Source: CAD feature listing. Evaluate the final solid. Frame: model axes, mm. Coordinates: 2 decimals unless noted, no trailing zeros. Write each loop counter-clockwise with the first axis right and the second up, starting at its lowest first coordinate (ties: lowest second). Pieces come first, ordered by that corner, then holes. Notation, with made-up numbers: M 21.25,-17.75 L 31.25,-17.75 A14 cw 31.25,7.25 Z; hole C 65.25,-20 d8. An arc over 180 degrees is marked long. One line per item, written item: value. Start each with the question number.
Item 1: Mould query, pull axis Z, two halves, no side actions, for faces 1 (the flat face through (7, 3, -1.9)), 2 (the flat face through (60, 3, 0)), 3 (the flat face through (94, 3, -6.1)). Classes: released by +Z, released by -Z, zero draft, split by the parting line, or undercut.
Item 2: Cut plane D-D, the plane x = 58. Output: boundary loops of the cut face in (y, z), then the cut area to 3 significant figures.
Item 3: Cut plane B-B, the plane z = -115. Output: boundary loops of the cut face in (x, y).
Item 4: Ray query, L1, parallel to Z at x = 43, y = 3.85; L2, parallel to Z at x = 106.2, y = 2.45; L3, parallel to X at y = 4.75, z = -115. Return the intervals inside material, ascending. Write a range as from..to.
Item 5: Pin query (flat end, axial travel): P1, Ø3, axis at x = 57.5, z = -30.5, coming from the +Y side. Return the tip coordinate at first contact, or that it passes through.
Item 6: Cut plane C-C, the plane z = -31.5. Output: boundary loops of the cut face in (x, y), then the cut area to 3 significant figures.
Item 7: Cut plane A-A, the plane x = 15.2. Output: boundary loops of the cut face in (y, z).
```python
from build123d import *

# Parameters (mm, degrees)
SKETCH_1_W          = 121.4
SKETCH_1_H          = 128.7
EXTRUDE_1_DEPTH     = 1.5
EXTRUDE_2_DEPTH     = 2
SKETCH_3_W          = 1.5
SKETCH_3_H          = 96.8
SKETCH_3_W_2        = 113.8
SKETCH_3_H_2        = 1.5
EXTRUDE_3_DEPTH     = 2
SKETCH_5_W          = 121.4
SKETCH_5_H          = 8
SKETCH_5_W_2        = 32.9
SKETCH_5_H_2        = 4.2
SKETCH_5_W_3        = 48
EXTRUDE_5_DEPTH     = 4
SKETCH_7_R          = 4.75
EXTRUDE_10_DEPTH    = 4
SKETCH_8_R          = 1.75
CUT_EXTRUDE_3_DEPTH = 5.5
CHAMFER_1_SIZE      = 1.6
SKETCH_10_W         = 48
SKETCH_10_H         = 6.1
CUT_EXTRUDE_4_DEPTH = 4
CHAMFER_2_SIZE      = 0.5
CHAMFER_2_SIZE2     = 0.866025404


with BuildPart() as part:
    # Эскиз1 → Бобышка-Вытянуть1 (new body)
    with BuildSketch(Plane(origin=(0, 0, 0), x_dir=(1, 0, 0), z_dir=(0, 1, 0))):
        with Locations((60.7, 64.35)):
            Rectangle(SKETCH_1_W, SKETCH_1_H)
    extrude(amount=EXTRUDE_1_DEPTH)

    # Эскиз2 → Бобышка-Вытянуть2 (add)
    with BuildSketch(Plane(origin=(0, 1.5, 0), x_dir=(1, 0, 0), z_dir=(0, 1, 0))):
        Polygon((0, 8), (0, 128.7), (121.4, 128.7), (121.4, 8), (117.6, 8), (117.6, 124.9), (3.8, 124.9), (3.8, 8), align=None)
    extrude(amount=EXTRUDE_2_DEPTH)

    # Эскиз3 → Бобышка-Вытянуть3 (add)
    with BuildSketch(Plane(origin=(0, 3.5, 0), x_dir=(1, 0, 0), z_dir=(0, 1, 0))):
        Polygon((0, 8), (3.8, 8), (3.8, 124.9), (117.6, 124.9), (117.6, 8), (121.4, 8), (121.4, 128.7), (0, 128.7), align=None)
        with Locations((1.85, 59)):
            Rectangle(SKETCH_3_W, SKETCH_3_H, mode=Mode.SUBTRACT)
        with Locations((60.7, 126.85)):
            Rectangle(SKETCH_3_W_2, SKETCH_3_H_2, mode=Mode.SUBTRACT)
        with Locations((119.55, 59)):
            Rectangle(SKETCH_3_W, SKETCH_3_H, mode=Mode.SUBTRACT)
    extrude(amount=EXTRUDE_3_DEPTH)

    # Эскиз5 → Бобышка-Вытянуть5 (add)
    with BuildSketch(Plane(origin=(0, 1.5, 0), x_dir=(1, 0, 0), z_dir=(0, 1, 0))):
        with Locations((60.7, 4)):
            Rectangle(SKETCH_5_W, SKETCH_5_H)
        with Locations((18.35, 4)):
            Rectangle(SKETCH_5_W_2, SKETCH_5_H_2, mode=Mode.SUBTRACT)
        with Locations((103.05, 4)):
            Rectangle(SKETCH_5_W_2, SKETCH_5_H_2, mode=Mode.SUBTRACT)
        with Locations((60.7, 4)):
            Rectangle(SKETCH_5_W_3, SKETCH_5_H_2, mode=Mode.SUBTRACT)
    extrude(amount=EXTRUDE_5_DEPTH)

    # Эскиз7 → Бобышка-Вытянуть10 (add)
    with BuildSketch(Plane(origin=(0, 1.5, 0), x_dir=(1, 0, 0), z_dir=(0, 1, 0))):
        with Locations((5.95, 115)):
            Circle(SKETCH_7_R)
        with Locations((115.45, 115)):
            Circle(SKETCH_7_R)
        with Locations((15.2, 4.75)):
            Circle(SKETCH_7_R)
        with Locations((106.2, 4.75)):
            Circle(SKETCH_7_R)
    extrude(amount=EXTRUDE_10_DEPTH)

    # Эскиз8 → Вырез-Вытянуть3 (cut)
    with BuildSketch(Plane.XZ):
        with Locations(Location((15.2, -4.75, 0), (0, 0, 270))):
            Circle(SKETCH_8_R)
        with Locations(Location((106.2, -4.75, 0), (0, 0, 270))):
            Circle(SKETCH_8_R)
        with Locations(Location((5.95, -115, 0), (0, 0, 270))):
            Circle(SKETCH_8_R)
        with Locations(Location((115.45, -115, 0), (0, 0, 270))):
            Circle(SKETCH_8_R)
    extrude(amount=-CUT_EXTRUDE_3_DEPTH, mode=Mode.SUBTRACT)

    # Фаска1
    chamfer_1_edges = [part.edges().sort_by_distance(p)[0] for p in [
        (115.45, 0, -113.25),
        (5.95, 0, -113.25),
        (106.2, 0, -3),
        (15.2, 0, -3),
    ]]
    chamfer(chamfer_1_edges, length=CHAMFER_1_SIZE)

    # Эскиз10 → Вырез-Вытянуть4 (cut)
    with BuildSketch(Plane(origin=(0, 5.5, 0), x_dir=(1, 0, 0), z_dir=(0, 1, 0))):
        with Locations((60.7, 4.95)):
            Rectangle(SKETCH_10_W, SKETCH_10_H)
    extrude(amount=-CUT_EXTRUDE_4_DEPTH, mode=Mode.SUBTRACT)

    # Фаска2
    chamfer_2_edges = [part.edges().sort_by_distance(p)[0] for p in [
        (0, 0, -64.35),
        (60.7, 0, -128.7),
        (121.4, 0, -64.35),
        (60.7, 0, 0),
    ]]
    chamfer_2_side = [part.faces().sort_by_distance(p)[0] for p in [
        (60.7, 0, -64.390759898),
    ]]
    chamfer(chamfer_2_edges, length=CHAMFER_2_SIZE, length2=CHAMFER_2_SIZE2, reference=chamfer_2_side[0])


solid = part.part
```
From the geometry:
1. face 1: undercut
1. face 2: released by +Z
1. face 3: undercut
2. outline: M 0,-128.2 L 0.87,-128.7 L 5.5,-128.7 L 5.5,-127.6 L 3.5,-127.6 L 3.5,-126.1 L 5.5,-126.1 L 5.5,-124.9 L 1.5,-124.9 L 1.5,-1.9 L 5.5,-1.9 L 5.5,0 L 0.87,0 L 0,-0.5 Z
2. area: 212 mm²
3. outline: M 0,0.87 L 0.5,0 L 2.6,0 L 4.2,1.6 L 4.2,5.5 L 0,5.5 Z; M 7.7,1.6 L 9.3,0 L 112.1,0 L 113.7,1.6 L 113.7,5.5 L 110.7,5.5 L 110.7,1.5 L 10.7,1.5 L 10.7,5.5 L 7.7,5.5 Z; M 117.2,1.6 L 118.8,0 L 120.9,0 L 121.4,0.87 L 121.4,5.5 L 117.2,5.5 Z
4. L1: z = -128.7..-127.6, -126.1..-124.9, -1.9..0
4. L2: z = -128.7..-124.9, -9.5..-6.5, -3..0
4. L3: x = 0..4.2, 7.7..10.7, 110.7..113.7, 117.2..121.4
5. P1: stops at y = 1.5
6. outline: M 0,0.87 L 0.5,0 L 120.9,0 L 121.4,0.87 L 121.4,5.5 L 120.3,5.5 L 120.3,3.5 L 118.8,3.5 L 118.8,5.5 L 117.6,5.5 L 117.6,1.5 L 3.8,1.5 L 3.8,5.5 L 2.6,5.5 L 2.6,3.5 L 1.1,3.5 L 1.1,5.5 L 0,5.5 Z
6. area: 206 mm²
7. outline: M 0,-128.2 L 0.87,-128.7 L 5.5,-128.7 L 5.5,-127.6 L 3.5,-127.6 L 3.5,-126.1 L 5.5,-126.1 L 5.5,-124.9 L 1.5,-124.9 L 1.5,-9.5 L 5.5,-9.5 L 5.5,-6.5 L 1.6,-6.5 L 0,-8.1 Z; M 0,-1.4 L 1.6,-3 L 5.5,-3 L 5.5,0 L 0.87,0 L 0,-0.5 Z
